For this review, take the finished solid that the model builds, in its own axes (mm). A direction names the side the tool comes from. Coordinates: 2 decimals unless noted, no trailing zeros. Order: outer loops, then holes, each group sorted by start corner. A loop starts at its lowest first (then second) coordinate and runs counter-clockwise, first axis right, second up. Notation, with made-up numbers: (-4.75, 12) -> (17.25, 12) arc R25 ccw to (17.25, 40) -> close; hole circle Ø1 at (-14, -22.5). An arc over 180 degrees is marked (long way). Return JSON: item names as keys, results as strings. Group by question number.
Item 1: Machinability: for faces 1 (the flat face through (30, -14, 12)), 2 (the cylindrical face through (8.113, -10.727, 14.114)), 3 (the cylindrical face through (34.358, -14.032, 8.451)), 4 (the flat face through (8, -27.9, 11)), 5 (the flat face through (1, 30, 2)), which of the approach directions +Z, -Z, +X, -X, +Y, -Y give a long, thin tool a straight path to every point of the face, cutting with its end or side? Answer none if there is none.
Item 2: Take a section at A-A (x = 8.5). Write out the cut boundary in (y, z).
Item 3: Take a section at C-C (y = 11). Write out the cut boundary in (x, z).
Item 4: Take a section at D-D (x = -17). Write out the cut boundary in (y, z).
Item 5: For line 1 along Y through (x, z) = (-0.5, 7.5); line 2 along Y through (x, z) = (21, 7.75); line 3 along Z through (x, y) = (-6, -11), list the stretches that pass through material, from the lowest coordinate up.
Item 6: Insertion check: pin 1 (4 mm diameter, centred on x = -11, y = 4.5, fed in from +Z); pin 2 (8 mm diameter, centred on y = 5.5, z = 9.5, fed in from -X); pin 3 (8 mm diameter, centred on x = 11.5, z = 16, fed in from -Y). Each pin has a flat end and moves straight along its axis. Give the tip position at first contact, or say it passes through.
Item 7: Take a section at B-B (z = 13.25). Write out the cut boundary in (x, y), then the cut area to 3 significant figures.
Item 8: Draft analysis for pull direction Y (two halves, no side actions). For faces 6 (the flat face through (8, -23.4, 11)), 7 (the cylindrical face through (-24.035, 18.605, 8.451)), 8 (the flat face through (8, -23.2, 15)), 9 (the flat face through (40, -2, 2)), state which applies: +Y half, -Y half, draft (parallel to the pull), parting line (faces both ways), or undercut.
```python
from build123d import *

# Parameters (mm, degrees)
F2_DEPTH      = 5
F3_DEPTH      = 12
F6_START      = 23.4
F6_DEPTH      = 4.5
F7_DEPTH      = 23.2
F7_DEPTH_BACK = 2.1


with BuildPart() as f2:
    # F0 (on Top) → F2 (new body)
    with BuildSketch(Plane.XY):
        Polygon((-40, -33.5), (40, -33.5), (40, -32.5), (40, -30), (40, 30), (-40, 30), (-40, -30), (-40, -32.5), align=None)
    extrude(amount=F2_DEPTH)

    # F1 (on Top) → F3 (join)
    with BuildSketch(Plane.XY):
        with BuildLine():
            ThreePointArc((-2.6521374299, 16.6687909301), (-16.3807168127, 12.4606072464), (-30.1092961955, 16.6687909301))
            ThreePointArc((-30.1092961955, 16.6687909301), (-16.3807168127, 7.9968769917), (-2.6521374299, 16.6687909301))
        make_face()
        with BuildLine():
            ThreePointArc((-14.5791374299, 16.6687909301), (-16.3571438566, 15.9253940397), (-18.1821348298, 16.5445497046))
            ThreePointArc((-18.1821348298, 16.5445497046), (-24.124880914, 18.6067924142), (-30.1092961955, 16.6687909301))
            ThreePointArc((-30.1092961955, 16.6687909301), (-16.3807168127, 12.4606072464), (-2.6521374299, 16.6687909301))
            ThreePointArc((-2.6521374299, 16.6687909301), (-8.6156374299, 18.3140845418), (-14.5791374299, 16.6687909301))
        make_face()
        with BuildLine():
            Line((20.4430632293, -23.025110057), (20.4430632293, -27.6445335891))
            ThreePointArc((20.4430632293, -27.6445335891), (34.3612617995, -13.7263350189), (20.4430632293, 0.1918635513))
            Line((20.4430632293, 0.1918635513), (20.4430632293, -4.4275599807))
            ThreePointArc((20.4430632293, -4.4275599807), (29.7418382675, -13.7263350189), (20.4430632293, -23.025110057))
        make_face()
    extrude(amount=F3_DEPTH)

    # F5 (on Front) → F6 (join)
    with BuildSketch(Plane.XZ.offset(F6_START)):
        with BuildLine():
            Line((20.3935885802, 5.1095173694), (20.3935885802, 11.976900753))
            ThreePointArc((20.3935885802, 11.976900753), (4.5517351525, 20.8753907692), (-4.2704897933, 4.9909395166))
            Line((-4.2704897933, 4.9909395166), (14.5364608753, 5.0813579703))
            Line((14.5364608753, 5.0813579703), (20.3935885802, 5.1095173694))
        make_face()
    extrude(amount=F6_DEPTH)

    # F4 (on Front) → F7 (join, two sides)
    with BuildSketch(Plane.XZ) as f7_sk:
        with BuildLine():
            Line((20.3951951116, 5.0531513989), (20.3951951116, 11.9205347825))
            ThreePointArc((20.3951951116, 11.9205347825), (4.553341684, 20.8190247987), (-4.2688832618, 4.9345735461))
            Line((-4.2688832618, 4.9345735461), (1.6444845672, 4.9630033317))
            Line((1.6444845672, 4.9630033317), (1.5165806981, 5.4129436612))
            ThreePointArc((1.5165806981, 5.4129436612), (8.2922385909, 14.1107486492), (14.5380674067, 5.0249919998))
            Line((14.5380674067, 5.0249919998), (20.3951951116, 5.0531513989))
        make_face()
    extrude(amount=F7_DEPTH)
    extrude(f7_sk.sketch, amount=-F7_DEPTH_BACK)


solid = f2.part
```
Findings below:
{
 "1": {"face 1": "+Z, +X, +Y, -Y", "face 2": "+Y", "face 3": "+Z, +X", "face 4": "+Z, +X, -X, -Y", "face 5": "+Z, -Z, +X, -X, +Y"},
 "2": {"outline": "(-33.5, 0) -> (30, 0) -> (30, 5) -> (-33.5, 5) -> close; (-27.9, 5.05) -> (-23.4, 5.05) -> (-23.4, 21.35) -> (-27.9, 21.35) -> close; (-23.2, 14.1) -> (2.1, 14.1) -> (2.1, 21.3) -> (-23.2, 21.3) -> close"},
 "3": {"outline": "(-40, 0) -> (40, 0) -> (40, 5) -> (-7.31, 5) -> (-7.31, 12) -> (-25.45, 12) -> (-25.45, 5) -> (-40, 5) -> close"},
 "4": {"outline": "(-33.5, 0) -> (30, 0) -> (30, 5) -> (15.98, 5) -> (15.98, 12) -> (8.01, 12) -> (8.01, 5) -> (-33.5, 5) -> close"},
 "5": {"line 1": "y = -27.9 to -23.4, -23.2 to 2.1", "line 2": "y = -27.63 to -23.01, -4.44 to 0.18", "line 3": "z = 0 to 5"},
 "6": {"pin 1": "stops at z = 5", "pin 2": "stops at x = -22.97", "pin 3": "stops at y = -27.9"},
 "7": {"outline": "(-3.88, -27.9) -> (19.97, -27.9) -> (19.97, -23.4) -> (-3.88, -23.4) -> close; (-3.85, -23.2) -> (4.76, -23.2) -> (4.76, 2.1) -> (-3.85, 2.1) -> close; (11.41, -23.2) -> (19.95, -23.2) -> (19.95, 2.1) -> (11.41, 2.1) -> close", "area": "541 mm2"},
 "8": {"face 6": "undercut", "face 7": "+Y half", "face 8": "undercut", "face 9": "draft"}
}
